Build history of the part. All positions in model axes, mm. A direction names the side the tool comes from. Give positions to 0.01 mm unless a question says otherwise; leave off trailing zeros. Write each loop counter-clockwise with the first axis right and the second up, starting at its lowest first coordinate (ties: lowest second). Pieces come first, ordered by that corner, then holes. Notation, with made-up numbers: (24.25, 5) -> (70.25, 5) arc R23 ccw to (70.25, 37) -> close; hole circle Ø5 at (81, 7.5). An arc over 180 degrees is marked (long way). Put each result on its own line as item: value.
from build123d import *

# Parameters (mm, degrees)
SKETCH1_W                     = 175
SKETCH1_H                     = 125
SKETCH1_R                     = 2.75
BASE_FLANGE1_DEPTH            = 2
EDGE_FLANGE1_STRIP_W          = 12.06
EDGE_FLANGE1_STRIP_H          = 2
EDGE_FLANGE1_STRIP_CUT_DEPTH  = 175
EDGE_FLANGE1_DEPTH            = 175
EDGE_FLANGE3_STRIP_W          = 12.06
EDGE_FLANGE3_STRIP_H          = 2
EDGE_FLANGE3_STRIP_CUT_DEPTH  = 110
EDGE_FLANGE3_RELIEF_W         = 13.06
EDGE_FLANGE3_RELIEF_H         = 1
EDGE_FLANGE3_RELIEF_CUT_DEPTH = 2
EDGE_FLANGE3_DEPTH            = 110
CUT_EXTRUDE2_REACH            = 164.808
SKETCH18_R                    = 2.1
FILLET1_R                     = 5


# Sheet-metal steps are written as plain solids
with BuildPart() as part:
    # Sketch1 → Base-Flange1 (new body)
    with BuildSketch(Plane.XY):
        Rectangle(SKETCH1_W, SKETCH1_H)
        with Locations((70.5634, 45.5634)):
            Circle(SKETCH1_R, mode=Mode.SUBTRACT)
        with Locations((70.5634, -45.5634)):
            Circle(SKETCH1_R, mode=Mode.SUBTRACT)
        with Locations((-70.5634, 45.5634)):
            Circle(SKETCH1_R, mode=Mode.SUBTRACT)
        with Locations((-70.5634, -45.5634)):
            Circle(SKETCH1_R, mode=Mode.SUBTRACT)
    extrude(amount=BASE_FLANGE1_DEPTH)

    # Edge-Flange1 strip (across the edge) → Edge-Flange1 strip cut (cut)
    with BuildSketch(Plane(origin=(-87.5, -62.5, 2), x_dir=(0, 1, 0), z_dir=(1, 0, 0))):
        with Locations((-2, -1)):
            Rectangle(EDGE_FLANGE1_STRIP_W, EDGE_FLANGE1_STRIP_H)
    extrude(amount=EDGE_FLANGE1_STRIP_CUT_DEPTH, mode=Mode.SUBTRACT)

    # Edge-Flange1 section (across the edge) → Edge-Flange1 (add)
    with BuildSketch(Plane(origin=(-87.5, -62.5, 2), x_dir=(0, 1, 0), z_dir=(1, 0, 0))):
        with BuildLine():
            Line((0, 2.03), (0, 60))
            Line((0, 60), (2, 60))
            Line((2, 60), (2, 2.03))
            ThreePointArc((2, 2.03), (2.594573234, 0.594573234), (4.03, 0))
            Line((4.03, 0), (4.03, -2))
            ThreePointArc((4.03, -2), (1.180359672, -0.819640328), (0, 2.03))
        make_face()
    extrude(amount=EDGE_FLANGE1_DEPTH)

    # Edge-Flange3 strip (across the edge) → Edge-Flange3 strip cut (cut)
    with BuildSketch(Plane(origin=(87.5, -62.5, 62), x_dir=(0, 0, -1), z_dir=(-1, 0, 0))):
        with Locations((-2, -1)):
            Rectangle(EDGE_FLANGE3_STRIP_W, EDGE_FLANGE3_STRIP_H)
    extrude(amount=EDGE_FLANGE3_STRIP_CUT_DEPTH, mode=Mode.SUBTRACT)

    # Edge-Flange3 relief (on the sheet) → Edge-Flange3 relief cut (cut)
    with BuildSketch(Plane(origin=(87.5, -62.5, 57.97), x_dir=(0, 0, -1), z_dir=(0, -1, 0))):
        with Locations((-5.53, -110.5)):
            Rectangle(EDGE_FLANGE3_RELIEF_W, EDGE_FLANGE3_RELIEF_H)
    extrude(amount=-EDGE_FLANGE3_RELIEF_CUT_DEPTH, mode=Mode.SUBTRACT)

    # Edge-Flange3 section (across the edge) → Edge-Flange3 (add)
    with BuildSketch(Plane(origin=(87.5, -62.5, 62), x_dir=(0, 0, -1), z_dir=(-1, 0, 0))):
        with BuildLine():
            Line((0, 2.03), (0, 60))
            Line((0, 60), (2, 60))
            Line((2, 60), (2, 2.03))
            ThreePointArc((2, 2.03), (2.594573234, 0.594573234), (4.03, 0))
            Line((4.03, 0), (4.03, -2))
            ThreePointArc((4.03, -2), (1.180359672, -0.819640328), (0, 2.03))
        make_face()
    extrude(amount=EDGE_FLANGE3_DEPTH)

    # Sketch18 → Cut-Extrude2 (cut, up to next)
    with BuildSketch(Plane.XY.offset(62), mode=Mode.PRIVATE) as cut_extrude2_sk1:
        with Locations((-9, -71.372677549)):
            Circle(SKETCH18_R)
    cut_extrude2_tool1 = extrude(cut_extrude2_sk1.sketch, amount=-CUT_EXTRUDE2_REACH, mode=Mode.PRIVATE) & part.part
    # Sketch18 → Cut-Extrude2 (cut, up to next)
    with BuildSketch(Plane.XY.offset(62), mode=Mode.PRIVATE) as cut_extrude2_sk2:
        with Locations((-9, -113.627322451)):
            Circle(SKETCH18_R)
    cut_extrude2_tool2 = extrude(cut_extrude2_sk2.sketch, amount=-CUT_EXTRUDE2_REACH, mode=Mode.PRIVATE) & part.part
    # Sketch18 → Cut-Extrude2 (cut, up to next)
    with BuildSketch(Plane.XY.offset(62), mode=Mode.PRIVATE) as cut_extrude2_sk3:
        with Locations((74, -71.372677549)):
            Circle(SKETCH18_R)
    cut_extrude2_tool3 = extrude(cut_extrude2_sk3.sketch, amount=-CUT_EXTRUDE2_REACH, mode=Mode.PRIVATE) & part.part
    # Sketch18 → Cut-Extrude2 (cut, up to next)
    with BuildSketch(Plane.XY.offset(62), mode=Mode.PRIVATE) as cut_extrude2_sk4:
        with Locations((74, -113.627322451)):
            Circle(SKETCH18_R)
    cut_extrude2_tool4 = extrude(cut_extrude2_sk4.sketch, amount=-CUT_EXTRUDE2_REACH, mode=Mode.PRIVATE) & part.part
    add(cut_extrude2_tool1.solids().sort_by_distance((-9, -71.372678, 62))[0], mode=Mode.SUBTRACT)
    add(cut_extrude2_tool2.solids().sort_by_distance((-9, -113.627322, 62))[0], mode=Mode.SUBTRACT)
    add(cut_extrude2_tool3.solids().sort_by_distance((74, -71.372678, 62))[0], mode=Mode.SUBTRACT)
    add(cut_extrude2_tool4.solids().sort_by_distance((74, -113.627322, 62))[0], mode=Mode.SUBTRACT)

    # Fillet1
    fillet1_edges = [part.edges().sort_by_distance(p)[0] for p in [
        (-87.5, -61.5, 62),
        (87.5, 62.5, 1),
        (-87.5, 62.5, 1),
        (87.5, -122.5, 61),
        (-22.5, -122.5, 61),
    ]]
    fillet(fillet1_edges, radius=FILLET1_R)


solid = part.part
1) Pull direction Y, two halves, no side cores. Call faces 4 (the cylindrical face through (67.816, -45.442, 0.986)), 5 (the cylindrical face through (-21.07, -121, 60.99)), 6 (the cylindrical face through (-86.07, -61.49, 60.5)): released by +Y, released by -Y, zero draft, split by the parting line, or undercut.
Filled sheet:
face 4: undercut
face 5: released by -Y
face 6: zero draft
2) Wall check: L1, parallel to Y at x = -9, z = 60.6; L2, parallel to Y at x = -9, z = 61.2; L3, parallel to Z at x = 46.5, y = 37.5. Give the ranges that are in metal, low to high.
Filled sheet:
L1: -122.5 to -115.73, -111.53 to -73.47, -69.27 to -61.48
L2: -122.5 to -115.73, -111.53 to -73.47, -69.27 to -62.12
L3: 0 to 2
3) Slice it at C-C (z = 15.5). Write the cut outline in (x, y).
Filled sheet:
outline: (-87.5, -62.5) -> (87.5, -62.5) -> (87.5, -60.5) -> (-87.5, -60.5) -> close
4) Slice it at D-D (y = 9.5). Write the cut outline in (x, z).
Filled sheet:
outline: (-87.5, 0) -> (87.5, 0) -> (87.5, 2) -> (-87.5, 2) -> close
5) Pin check, flat tips, straight feed: pin 1 (3 mm diameter, centred on x = -9.5, z = 18, fed in from -Y); pin 2 (6.5 mm diameter, centred on x = -9, y = -71.37, fed in from +Z); pin 3 (4 mm diameter, centred on y = -91.5, z = 60.5, fed in from -X); pin 4 (7 mm diameter, centred on x = 70.56, y = -45.56, fed in from +Z). Stop position of each tip, or through.
Filled sheet:
pin 1: y = -62.5
pin 2: z = 62
pin 3: x = -22.5
pin 4: z = 2
6) Slice it at B-B (x = 26). Write the cut outline in (y, z).
Filled sheet:
outline: (-122.5, 60) -> (-64.53, 60) arc R2.03 cw to (-62.5, 57.97) -> (-62.5, 4.03) arc R4.03 ccw to (-58.47, 0) -> (62.5, 0) -> (62.5, 2) -> (-58.47, 2) arc R2.03 cw to (-60.5, 4.03) -> (-60.5, 57.97) arc R4.03 ccw to (-64.53, 62) -> (-122.5, 62) -> close
7) Tool access for faces 1 (the flat face through (33, -94, 60)), 2 (the flat face through (-1, 3, 2)), 3 (the cylindrical face through (-10.548, -69.953, 61.014)): list every direction of +Z, -Z, +X, -X, +Y, -Y with a clear straight run to the whole face (end or side of a thin tool).
Filled sheet:
face 1: -Z, +X, -X, -Y
face 2: +Z, +X, -X, +Y
face 3: +Z, -Z
8) Slice it at A-A (x = -9). Write the cut outline in (y, z).
Filled sheet:
outline: (-122.5, 60) -> (-115.73, 60) -> (-115.73, 62) -> (-122.5, 62) -> close; (-111.53, 60) -> (-73.47, 60) -> (-73.47, 62) -> (-111.53, 62) -> close; (-69.27, 60) -> (-64.53, 60) arc R2.03 cw to (-62.5, 57.97) -> (-62.5, 4.03) arc R4.03 ccw to (-58.47, 0) -> (62.5, 0) -> (62.5, 2) -> (-58.47, 2) arc R2.03 cw to (-60.5, 4.03) -> (-60.5, 57.97) arc R4.03 ccw to (-64.53, 62) -> (-69.27, 62) -> close
